from build123d import *
from build123d import SkipClean  # not in build123d's __all__

# Parameters (mm, degrees)
F1_DEPTH = 6.35
F2_R     = 3.4925
F3_DEPTH = 6.35
F4_W     = 33.274
F4_H     = 6.35
F5_DEPTH = 9.08304
F6_W     = 5.08
F6_H     = 6.35
F7_DEPTH = 11.7348
F8_R     = 1.016
F9_DEPTH = 6.35


# Not quite as in the source:
# - after a boolean that leaves OpenCascade's solid faulty, fix() repairs it


with BuildPart() as f1:
    # F0 (on Right) → F1 (new body)
    with BuildSketch(Plane.YZ):
        with BuildLine():
            Line((0, -6.35), (0, 0))
            Line((0, 0), (-32.766, 0))
            Line((-32.766, 0), (-35.2239654818, 0))
            Line((-35.2239654818, 0), (-37.4816982729, -2.0558894312))
            Line((-37.4816982729, -2.0558894312), (-37.2950388694, -7.1750314139))
            ThreePointArc((-37.2950388694, -7.1750314139), (-38.2710574955, -9.7264527612), (-40.7852194514, -10.7947939567))
            Line((-40.7852194514, -10.7947939567), (-49.3363048096, -10.7947939567))
            Line((-49.3363048096, -10.7947939567), (-75.565, -34.67862))
            Line((-75.565, -34.67862), (-75.565, -48.67862))
            Line((-75.565, -48.67862), (-56.515, -48.67862))
            Line((-56.515, -48.67862), (-56.515, -25.1183178527))
            Line((-56.515, -25.1183178527), (-46.3639643027, -15.8747939567))
            Line((-46.3639643027, -15.8747939567), (-35.5806867418, -15.8747939567))
            Line((-35.5806867418, -15.8747939567), (-32.766, -13.3117427633))
            Line((-32.766, -13.3117427633), (-32.766, -6.35))
            Line((-32.766, -6.35), (0, -6.35))
        make_face()
        with BuildLine():
            ThreePointArc((-69.54, -44.67862), (-72.04, -39.67862), (-69.54, -34.67862))
            Line((-69.54, -34.67862), (-62.54, -34.67862))
            ThreePointArc((-62.54, -34.67862), (-60.04, -39.67862), (-62.54, -44.67862))
            Line((-62.54, -44.67862), (-69.54, -44.67862))
        make_face(mode=Mode.SUBTRACT)
    extrude(amount=F1_DEPTH)

    # F2 (on face) → F3 (join)
    with BuildSketch(Plane.YZ.offset(6.35)):
        Polygon((-32.766, -13.3117427633), (-32.766, 0), (-46.3639643027, 0), (-49.3577194514, -2.9937551487), (-49.3577194514, -12.8810388079), (-46.3639643027, -15.8747939567), (-35.5806867418, -15.8747939567), align=None)
        with Locations((-40.7852194514, -7.3022939567)):
            Circle(F2_R, mode=Mode.SUBTRACT)
    with SkipClean():  # cleaning this boolean's faces spoils the solid; the shape is the same uncleaned
        extrude(amount=F3_DEPTH)

    # F4 (on face) → F5 (join)
    with BuildSketch(Plane.YZ.offset(6.35)):
        with Locations((-16.637, -3.175)):
            Rectangle(F4_W, F4_H)
    extrude(amount=F5_DEPTH)

    add(f1.part.fix(), mode=Mode.REPLACE)

    # F6 (on face) → F7 (join)
    with BuildSketch(Plane.YZ.offset(15.43304)):
        with Locations((-2.54, -3.175)):
            Rectangle(F6_W, F6_H)
        with Locations((-30.734, -3.175)):
            Rectangle(F6_W, F6_H)
    extrude(amount=F7_DEPTH)

    add(f1.part.fix(), mode=Mode.REPLACE)

    # F8 (on face) → F9 (cut, through all)
    with BuildSketch(Plane.XY):
        with Locations((21.30044, -30.734)):
            Circle(F8_R)
        with Locations((21.30044, -2.54)):
            Circle(F8_R)
    extrude(amount=-F9_DEPTH, mode=Mode.SUBTRACT)


solid = f1.part
Can you work these out from the model? Positions are in its coordinate system, mm. A direction names the side the tool comes from. Give positions to 0.01 mm unless a question says otherwise; leave off trailing zeros. Loops run counter-clockwise (first coordinate to the right, second up) from the corner with the lowest first, then second, coordinate; pieces in that order, holes last. Notation, with made-up numbers: M 79,28 L 132,28 A22 ccw 132,54 Z; hole C 29.5,45 d11. An arc over 180 degrees is marked long. One line per item, written item: value.
1) I'm going to push flat-ended pins straight in: pin 1 (3 mm diameter, centred on x = 4, y = -46, fed in from +Z); pin 2 (8.5 mm diameter, centred on x = 6.5, y = -38.5, fed in from -Z); pin 3 (5 mm diameter, centred on x = 21.5, z = -3.5, fed in from -Y). Where does each tip first touch, or does it pass through?
Geometry check:
pin 1: stops at z = -10.79
pin 2: stops at z = -15.87
pin 3: stops at y = -33.27
2) On a 3-axis mill with a long thin cutter (end or side, diameter ignored), from which of +Z, -Z, +X, -X, +Y, -Y can I reach the whole of each face in a straight line? I mean faces 1 (the face through (3.13, -72.04, -39.76)), 2 (the face through (3, -56.515, -37)), 3 (the face through (3.13, -37.39, -4.58)), 4 (the face through (15.433, -17, -3)), 5 (the face through (13, 0, -3)). Say none if no direction works.
Geometry check:
face 1: +X, -X
face 2: -Z, +X, -X, +Y
face 3: -X, -Y
face 4: +Z, -Z, +X
face 5: +Z, -Z, +X, -X, +Y
3) Imagine slicing it at A-A on y = -2.54. Write out the boundary of the cut face in (x, z).
Geometry check:
outline: M 0,-6.35 L 20.28,-6.35 L 20.28,0 L 0,0 Z; M 22.32,-6.35 L 27.17,-6.35 L 27.17,0 L 22.32,0 Z
4) Imagine slicing it at C-C on z = -29. Write out the boundary of the cut face in (x, y) (3 decimals), and give its area (3 significant figures).
Geometry check:
outline: M 0,-69.329 L 6.35,-69.329 L 6.35,-56.515 L 0,-56.515 Z
area: 81.4 mm²
5) Thinking about a two-plate mould opening in X: for faces 6 (the face through (20.285, -2.495, -3.131)), 7 (the face through (0, -46, -15)), 8 (the face through (9.48, -47.88, -14.36)), which applies, +X half, -X half, draft (parallel to the pull), parting line (faces both ways), or undercut?
Geometry check:
face 6: undercut
face 7: -X half
face 8: draft
6) Imagine slicing it at D-D on y = -67.5. Write out the boundary of the cut face in (x, z), and give its area (3 significant figures).
Geometry check:
outline: M 0,-48.68 L 6.35,-48.68 L 6.35,-44.68 L 0,-44.68 Z; M 0,-34.68 L 6.35,-34.68 L 6.35,-27.33 L 0,-27.33 Z
area: 72.0 mm²
7) Please list where these lines run through material, in increasing order: line 1 (Y direction, x = 20.75, z = -2.5); line 2 (Y direction, x = 3, z = -7.5); line 3 (Z direction, x = 9.75, y = -11.5).
Geometry check:
line 1: y = -33.27 to -31.59, -29.88 to -28.19, -5.08 to -3.39, -1.69 to 0
line 2: y = -37.3 to -32.77
line 3: z = -6.35 to 0
8) Imagine slicing it at B-B on y = -15. Write out the boundary of the cut face in (x, z), and give its area (3 significant figures).
Geometry check:
outline: M 0,-6.35 L 15.43,-6.35 L 15.43,0 L 0,0 Z
area: 98.0 mm²
